```python
from build123d import *

# Parameters (mm, degrees)
F0_W     = 199.39
F0_H     = 38.1
F1_DEPTH = 184.15
F2_W     = 19.05
F2_H     = 184.15
F3_DEPTH = 25.4
F4_R     = 2.286
F5_DEPTH = 25.4
F6_SIZE  = 2.54
F7_T     = -2.54


with BuildPart() as f1:
    # F0 (on Top) → F1 (new body)
    with BuildSketch(Plane.XY):
        with Locations((99.695, 19.05)):
            Rectangle(F0_W, F0_H)
    extrude(amount=F1_DEPTH)

    # F2 (on face) → F3 (join)
    with BuildSketch(Plane(origin=(0, 0, 0), x_dir=(0, -1, 0), z_dir=(-1, 0, 0))):
        with Locations((-9.525, 92.075)):
            Rectangle(F2_W, F2_H)
    extrude(amount=F3_DEPTH)

    # F4 (on face) → F5 (cut)
    with BuildSketch(Plane(origin=(0, 19.05, 0), x_dir=(-1, 0, 0), z_dir=(0, 1, 0))):
        with Locations((11.8618, 158.75)):
            Circle(F4_R)
        with Locations((11.8618, 133.35)):
            Circle(F4_R)
        with Locations((11.8618, 107.95)):
            Circle(F4_R)
        with Locations((11.8618, 82.55)):
            Circle(F4_R)
        with Locations((11.8618, 57.15)):
            Circle(F4_R)
        with Locations((11.8618, 31.75)):
            Circle(F4_R)
    extrude(amount=-F5_DEPTH, mode=Mode.SUBTRACT)

    # F6
    f6_edges = [f1.edges().sort_by_distance(p)[0] for p in [
        (-9.5758, 0, 158.75),
        (-9.5758, 0, 133.35),
        (-9.5758, 0, 107.95),
        (-9.5758, 0, 82.55),
        (-9.5758, 0, 57.15),
        (-9.5758, 0, 31.75),
    ]]
    chamfer(f6_edges, length=F6_SIZE)

    # F7
    f7_openings = [f1.faces().sort_by_distance(p)[0] for p in [
        (88.054654, 0, 92.040967),
    ]]
    offset(amount=F7_T, openings=f7_openings, kind=Kind.INTERSECTION)


solid = f1.part
```
Can you work these out from the model? Positions are in its coordinate system, mm. A direction names the side the tool comes from. Give positions to 0.01 mm unless a question says otherwise; leave off trailing zeros. Write each loop counter-clockwise with the first axis right and the second up, starting at its lowest first coordinate (ties: lowest second). Pieces come first, ordered by that corner, then holes. Notation, with made-up numbers: (72.5, 67) - (124.5, 67) arc R11 cw to (124.5, 75) - close; hole circle Ø10 at (-33, -16.5). An arc over 180 degrees is marked (long way). Write item = value, one per line. Start each with the question number.
1. Imagine slicing it at B-B (y = 24.5). Please give me the cut outline in (x, z).
2. On a 3-axis mill with a long thin cutter (end or side, diameter ignored), from which of +Z, -Z, +X, -X, +Y, -Y can I reach the whole of each face in a straight line? I mean faces 4 (the face through (196.85, 18, 91)), 5 (the face through (-12.917, 10.911, 131.322)), 6 (the face through (-14.456, 10.141, 86.619)). Say none if no direction works.
3. Imagine slicing it at C-C (x = 118.5). Please give me the cut outline in (y, z).
4. Imagine slicing it at A-A (z = 14). Please give me the cut outline in (x, y).
5. For pin 1 (15 mm diameter, centred on y = 32.5, z = 135.5, fed in from -X); pin 2 (2.5 mm diameter, centred on x = -11.86, z = 133.35, fed in from +Y); pin 3 (6 mm diameter, centred on x = -11.86, z = 57.15, fed in from +Y); pin 4 (7.5 mm diameter, centred on x = -11.86, z = 107.95, fed in from -Y), each with a flat end and sliding along its axis, tell me the tip position at first contact or that it passes through.
6. Thinking about a two-plate mould opening in Y: for faces 1 (the face through (89, 19, 0)), 2 (the face through (-14.09, 10.14, 154.47)), 3 (the face through (-15.5, 0, 35.4)), which applies, released by +Y, released by -Y, zero draft, split by the parting line, or undercut?
7. Please list where these lines run through material, in increasing order: line 1 (X direction, y = 11, z = 57); line 2 (X direction, y = 11, z = 71); line 3 (Z direction, x = 58, y = 20.5).
Worked answers:
q1.outline = (0, 0) - (199.39, 0) - (199.39, 184.15) - (0, 184.15) - close; hole (2.54, 2.54) - (196.85, 2.54) - (196.85, 181.61) - (2.54, 181.61) - close
q2.face_4 = -Y
q2.face_5 = +Y, -Y
q2.face_6 = none
q3.outline = (0, 0) - (38.1, 0) - (38.1, 184.15) - (0, 184.15) - (0, 181.61) - (35.56, 181.61) - (35.56, 2.54) - (0, 2.54) - close
q4.outline = (-25.4, 0) - (-22.86, 0) - (-22.86, 16.51) - (2.54, 16.51) - (2.54, 35.56) - (196.85, 35.56) - (196.85, 0) - (199.39, 0) - (199.39, 38.1) - (0, 38.1) - (0, 19.05) - (-25.4, 19.05) - close
q5.pin_1 = 0
q5.pin_2 = through
q5.pin_3 = 19.05
q5.pin_4 = 1.07
q6.face_1 = zero draft
q6.face_2 = undercut
q6.face_3 = released by -Y
q7.line_1 = -25.4 to -22.86, -16.69 to -14.14, -9.58 to -7.04, 196.85 to 199.39
q7.line_2 = -25.4 to -22.86, 196.85 to 199.39
q7.line_3 = 0 to 2.54, 181.61 to 184.15
